Read the model definition and answer for the solid it produces. Units are mm, in the model's axes. Give positions to 0.01 mm unless a question says otherwise; leave off trailing zeros. Order: outer loops, then holes, each group sorted by start corner. A loop starts at its lowest first (then second) coordinate and runs counter-clockwise, first axis right, second up.
```python
from build123d import *

# Parameters (mm, degrees)
F0_W     = 81
F0_H     = 15
F0_R     = 2.5
F0_H_2   = 30
F1_DEPTH = 4.9
F2_R     = 5
F3_R     = 5
F4_SIZE  = 2


with BuildPart() as f1:
    # F0 (on Top) → F1 (new body)
    with BuildSketch(Plane.XY):
        with Locations((1.9929800031, 0)):
            Rectangle(F0_W, F0_H)
        with Locations((-31.0070199969, 0)):
            Circle(F0_R, mode=Mode.SUBTRACT)
        with Locations((34.9929800031, 0)):
            Circle(F0_R, mode=Mode.SUBTRACT)
        with Locations((1.9929800031, -22.5)):
            Rectangle(F0_W, F0_H_2)
        with Locations((-31.0070199969, -30)):
            Circle(F0_R, mode=Mode.SUBTRACT)
        with Locations((34.9929800031, -30)):
            Circle(F0_R, mode=Mode.SUBTRACT)
    extrude(amount=F1_DEPTH)

    # F2
    f2_edges = [f1.edges().sort_by_distance(p)[0] for p in [
        (42.49298, 7.5, 2.45),
        (-38.50702, 7.5, 2.45),
    ]]
    fillet(f2_edges, radius=F2_R)

    # F3
    f3_edges = [f1.edges().sort_by_distance(p)[0] for p in [
        (42.49298, -37.5, 2.45),
        (-38.50702, -37.5, 2.45),
    ]]
    fillet(f3_edges, radius=F3_R)

    # F4
    f4_edges = [f1.edges().sort_by_distance(p)[0] for p in [
        (32.49298, 0, 4.9),
        (32.49298, -30, 4.9),
        (-33.50702, 0, 4.9),
        (-33.50702, -30, 4.9),
    ]]
    chamfer(f4_edges, length=F4_SIZE)


solid = f1.part
```
1) For a pull along X with two mould halves and no side action, classify faces 1 (the face through (-37.08, -36, 2.48)), 2 (the face through (1, -15, 4.9)), 3 (the face through (36.337, -27.892, 1.43)) as released by +X, released by -X, zero draft, split by the parting line, or undercut.
Final values:
face 1: released by -X
face 2: zero draft
face 3: undercut
2) Given pin 1 (8 mm diameter, centred on x = 34.99, y = -30, fed in from +Z); pin 2 (6.5 mm diameter, centred on x = -31.01, y = -30, fed in from +Z), each flat-ended and moving along its own axis, determine where each tip first touches the part or whether it passes through.
Final values:
pin 1: stops at z = 4.4
pin 2: stops at z = 3.65
3) The part is cut by section A-A on y = 0. Determine the outline of the cut face in (x, z).
Final values:
outline: (-38.51, 0) - (-33.51, 0) - (-33.51, 2.9) - (-35.51, 4.9) - (-38.51, 4.9) - close; (-28.51, 0) - (32.49, 0) - (32.49, 2.9) - (30.49, 4.9) - (-26.51, 4.9) - (-28.51, 2.9) - close; (37.49, 0) - (42.49, 0) - (42.49, 4.9) - (39.49, 4.9) - (37.49, 2.9) - close
4) Consider L1, parallel to Y at x = 34, z = 1; L2, parallel to X at y = 0.5, z = 2.5; L3, parallel to Y at x = 37, z = 2.2. Determine where each line is inside the solid, lowest interval first.
Final values:
L1: y = -37.5 to -32.29, -27.71 to -2.29, 2.29 to 7.5
L2: x = -38.51 to -33.46, -28.56 to 32.54, 37.44 to 42.49
L3: y = -37.5 to -31.49, -28.51 to -1.49, 1.49 to 7.5
5) The part is cut by section B-B on z = 1.2. Determine the outline of the cut face in (x, y).
Final values:
outline: (-38.51, -32.5) arc R5 ccw to (-33.51, -37.5) - (37.49, -37.5) arc R5 ccw to (42.49, -32.5) - (42.49, 2.5) arc R5 ccw to (37.49, 7.5) - (-33.51, 7.5) arc R5 ccw to (-38.51, 2.5) - close; hole circle Ø5 at (-31.01, -30); hole circle Ø5 at (-31.01, 0); hole circle Ø5 at (34.99, -30); hole circle Ø5 at (34.99, 0)
